For this review, take the finished solid that the model builds, in its own axes (mm). A direction names the side the tool comes from. Coordinates: 2 decimals unless noted, no trailing zeros. Loops run counter-clockwise (first coordinate to the right, second up) from the corner with the lowest first, then second, coordinate; pieces in that order, holes last.
```python
from build123d import *

# Parameters (mm, degrees)
BOSS_EXTRUDE1_DEPTH = 50.8
SKETCH3_R           = 2.4892
CUT_EXTRUDE1_DEPTH  = 54.975
SKETCH4_R           = 3.175
CUT_EXTRUDE2_DEPTH  = 2.5875


with BuildPart() as part:
    # Sketch2 → Boss-Extrude1 (new body)
    with BuildSketch(Plane.XY):
        Polygon((-1.5875, -1.5875), (100.0125, -1.5875), (100.0125, 0), (0, 0), (0, 50.8), (100.0125, 50.8), (100.0125, 52.3875), (-1.5875, 52.3875), align=None)
    extrude(amount=BOSS_EXTRUDE1_DEPTH)

    # Sketch3 → Cut-Extrude1 (cut, through all)
    with BuildSketch(Plane(origin=(0, 52.3875, 0), x_dir=(1, 0, 0), z_dir=(0, 1, 0))):
        with Locations((87.3125, -38.1)):
            Circle(SKETCH3_R)
        with Locations((87.3125, -12.7)):
            Circle(SKETCH3_R)
    extrude(amount=-CUT_EXTRUDE1_DEPTH, mode=Mode.SUBTRACT)

    # Sketch4 → Cut-Extrude2 (cut, through all)
    with BuildSketch(Plane(origin=(0, 0, 0), x_dir=(0, 0, -1), z_dir=(1, 0, 0))):
        with Locations((-25.4, 25.4)):
            Circle(SKETCH4_R)
    extrude(amount=-CUT_EXTRUDE2_DEPTH, mode=Mode.SUBTRACT)


solid = part.part
```
Q1. For pin 1 Ø15 at (y, z) = (28, 25.5) entering from +X, flat-tipped, find the tip position at first contact; note if it passes through.
Q2. Machinability: for faces 4 (the face through (50, 52.388, 25)), 5 (the face through (49, 50.8, 25)), which of the approach directions +Z, -Z, +X, -X, +Y, -Y give a long, thin tool a straight path to every point of the face, cutting with its end or side? Answer none if there is none.
Q3. Consider section B-B (z = 12.7). State the section outline as (x, y) points.
Q4. Consider section A-A (x = 22). State the section outline as (y, z) points, then the cut area to 3 significant figures.
Q5. Consider section C-C (z = 25.4). State the section outline as (x, y) points (1 decimal), then the cut area to 3 significant figures.
Q6. The part is to be moulded in two halves that separate along X. For faces 1 (the face through (-0.78, 26.35, 22.37)), 2 (the face through (89.612, 51.605, 39.053)), 3 (the face through (0, 31, 25)), say which applies: +X half, -X half, draft (parallel to the pull), parting line (faces both ways), or undercut.
Q7. Consider section D-D (y = 25.4). State the section outline as (x, z) points (1 decimal).
Q8. Wall thickness on probe 1 along Y at (x, z) = (14, 14.5); probe 2 along X at (y, z) = (52.05, 12.7); probe 3 along Y at (x, z) = (-0.65, 25.4) (1 decimal): over which ranges is each line inside the solid? List them lowest first.
Model answer:
1. pin 1: stops at x = 0
2. face 4: +Z, -Z, +X, -X, +Y
2. face 5: +Z, -Z, +X
3. outline: (-1.59, -1.59) - (84.82, -1.59) - (84.82, 0) - (0, 0) - (0, 50.8) - (84.82, 50.8) - (84.82, 52.39) - (-1.59, 52.39) - close; (89.8, -1.59) - (100.01, -1.59) - (100.01, 0) - (89.8, 0) - close; (89.8, 50.8) - (100.01, 50.8) - (100.01, 52.39) - (89.8, 52.39) - close
4. outline: (-1.59, 0) - (0, 0) - (0, 50.8) - (-1.59, 50.8) - close; (50.8, 0) - (52.39, 0) - (52.39, 50.8) - (50.8, 50.8) - close
4. area: 161 mm2
5. outline: (-1.6, -1.6) - (100, -1.6) - (100, 0) - (0, 0) - (0, 22.2) - (-1.6, 22.2) - close; (-1.6, 28.6) - (0, 28.6) - (0, 50.8) - (100, 50.8) - (100, 52.4) - (-1.6, 52.4) - close
5. area: 393 mm2
6. face 1: draft
6. face 2: undercut
6. face 3: +X half
7. outline: (-1.6, 0) - (0, 0) - (0, 22.2) - (-1.6, 22.2) - close; (-1.6, 28.6) - (0, 28.6) - (0, 50.8) - (-1.6, 50.8) - close
8. probe 1: y = -1.59 to 0, 50.8 to 52.39
8. probe 2: x = -1.59 to 84.82, 89.8 to 100.01
8. probe 3: y = -1.6 to 22.2, 28.6 to 52.4
